```python
from build123d import *

# Parameters (mm, degrees)
SKETCH1_W              = 43
SKETCH1_H              = 100
BASE_FLANGE1_DEPTH     = 1.5
SKETCHED_BEND1_DEPTH   = 43
SKETCHED_BEND1_2_DEPTH = 43
F_3_0MM_DOWEL_HOLE1_D  = 3


# Read off the part's stored shape, not the designer's step: Sketched Bend1
# Sheet-metal steps are written as plain solids
with BuildPart() as part:
    # Sketch1 → Base-Flange1 (new body)
    with BuildSketch(Plane.XY):
        with Locations((21.5, 50)):
            Rectangle(SKETCH1_W, SKETCH1_H)
    extrude(amount=-BASE_FLANGE1_DEPTH)

    # Sketched Bend1 outline → Sketched Bend1 (cut)
    with BuildSketch(Plane.YZ):
        with BuildLine():
            Line((100, 0), (70.944250946, 0))
            ThreePointArc((70.944250946, 0), (70.127591172, -1.086838938), (68.83242709, -1.5))
            Line((68.83242709, -1.5), (100, -1.5))
            Line((100, -1.5), (100, 0))
        make_face()
    extrude(amount=SKETCHED_BEND1_DEPTH, mode=Mode.SUBTRACT)

    # Sketched Bend1 2 outline → Sketched Bend1 2 (add)
    with BuildSketch(Plane.YZ):
        with BuildLine():
            Line((69.56902709, 29.56902709), (69.56902709, 0.7366))
            ThreePointArc((69.56902709, 0.7366), (69.353281945, 0.215745145), (68.83242709, 0))
            Line((68.83242709, 0), (70.944250946, 0))
            ThreePointArc((70.944250946, 0), (71.037612433, 0.363053267), (71.06902709, 0.7366))
            Line((71.06902709, 0.7366), (71.06902709, 29.56902709))
            Line((71.06902709, 29.56902709), (69.56902709, 29.56902709))
        make_face()
    extrude(amount=SKETCHED_BEND1_2_DEPTH)

    # Ø3.0mm Dowel Hole1 (through all)
    with Locations(Plane(origin=(-21.797673733, -43.188016106, -1.5), x_dir=(-0.9396926207859104, 0.34202014332566333, 0), z_dir=(0, 0, -1))):
        with Locations((-26.893032931, 71.71065686), (-14.67702886, 67.264394997)):
            Hole(F_3_0MM_DOWEL_HOLE1_D / 2)


solid = part.part
```
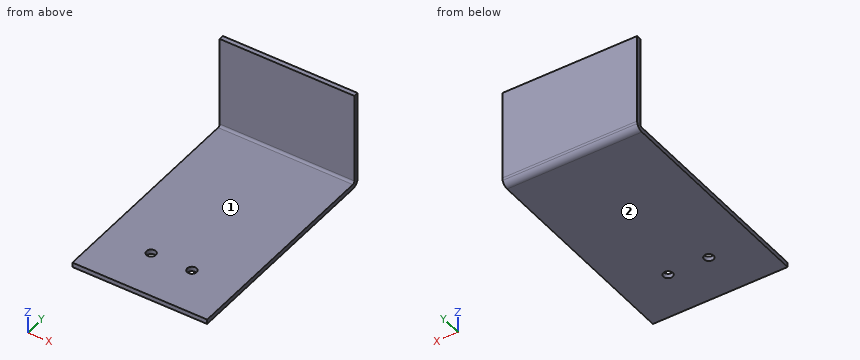
Source: CAD feature listing. Evaluate the final solid. Frame: model axes, mm. Face numbers are marked on the shaded views. A direction names the side the tool comes from. Coordinates: 2 decimals unless noted, no trailing zeros. Loops run counter-clockwise (first coordinate to the right, second up) from the corner with the lowest first, then second, coordinate; pieces in that order, holes last. Notation, with made-up numbers: M 89,59 L 142,59 A35 ccw 142,96 Z; hole C 26.25,77 d11. An arc over 180 degrees is marked long. Use a Markdown table: item, result. Add a question column.
Q1. Material intervals for L1, parallel to X at y = 15, z = -0.6; L2, parallel to Z at x = 27.5, y = 33; L3, parallel to Y at x = 23, z = 16.5, sorted ascending.
Q2. Section query D-D, the plane z = 18. Return loops of the section in (x, y), and give its area (3 significant figures).
Q3. Section query B-B, the plane x = 32. Return loops of the section in (y, z), and give its area (3 significant figures).
Q4. First-contact query: pin 1 (6 mm diameter, centred on x = 9.5, y = 45, fed in from +Z); pin 2 (1.8 mm diameter, centred on x = 28, y = 15, fed in from -Z); pin 3 (14.5 mm diameter, centred on x = 18.5, z = 9.5, fed in from -Y). Flat tips, straight axial feed; report the tip coordinate or a pass-through.
Q5. Section query A-A, the plane x = 15. Return loops of the section in (y, z), and give its area (4 significant figures).
Q6. Access query for the marked faces 1 and 2. Directions: +Z, -Z, +X, -X, +Y, -Y. A direction counts if a zero-diameter tool reaches every point of the face in a straight line with its end or side. Return the directions, or none.
Q7. Section query C-C, the plane y = 59. Return loops of the section in (x, z).
Result:
| question | item | result |
|---|---|---|
| 1 | L1 | x = 0 to 13.5, 16.5 to 26.5, 29.5 to 43 |
| 1 | L2 | z = -1.5 to 0 |
| 1 | L3 | y = 69.57 to 71.07 |
| 2 | outline | M 0,69.57 L 43,69.57 L 43,71.07 L 0,71.07 Z |
| 2 | area | 64.5 mm2 |
| 3 | outline | M 0,-1.5 L 68.83,-1.5 A2.24 ccw 71.07,0.74 L 71.07,29.57 L 69.57,29.57 L 69.57,0.74 A0.74 cw 68.83,0 L 0,0 Z |
| 3 | area | 150 mm2 |
| 4 | pin 1 | stops at z = 0 |
| 4 | pin 2 | passes through |
| 4 | pin 3 | stops at y = 69.57 |
| 5 | outline | M 0,-1.5 L 13.5,-1.5 L 13.5,0 L 0,0 Z; M 16.5,-1.5 L 68.83,-1.5 A2.24 ccw 71.07,0.74 L 71.07,29.57 L 69.57,29.57 L 69.57,0.74 A0.74 cw 68.83,0 L 16.5,0 Z |
| 5 | area | 145.5 mm2 |
| 6 | face 1 | +Z, +X, -X, -Y |
| 6 | face 2 | -Z, +X, -X, +Y, -Y |
| 7 | outline | M 0,-1.5 L 43,-1.5 L 43,0 L 0,0 Z |
